from build123d import *

# Parameters (mm, degrees)
PAD009_DEPTH    = 2.8
FILLET004_R     = 0.4
SKETCH025_W     = 12.7
SKETCH025_H     = 1.6
POCKET014_DEPTH = 2.801


with BuildPart() as part:
    # Sketch009 (on Face6 of ShapeBinder008) → Pad009 (new body)
    with BuildSketch(Plane.XZ.offset(60.388718)):
        with BuildLine():
            Line((37.8, 3.127675), (37.8, 0.327675))
            Line((37.8, 0.327675), (23.8, 0.327675))
            ThreePointArc((23.8, 0.327675), (23.4, -0.072325), (23.8, -0.472325))
            Line((23.8, -0.472325), (37.8, -0.472325))
            Line((37.8, -0.472325), (37.8, -33.872325))
            Line((37.8, -33.872325), (23.8, -33.872325))
            ThreePointArc((23.8, -33.872325), (23.4, -34.272325), (23.8, -34.672325))
            Line((23.8, -34.672325), (37.8, -34.672325))
            Line((37.8, -34.672325), (37.8, -37.472325))
            Line((37.8, -37.472325), (35.8, -38.222325))
            Line((35.8, -38.222325), (35.8, -37.472325))
            Line((35.8, -37.472325), (33, -37.472325))
            Line((33, -37.472325), (33, -39.472325))
            Line((33, -39.472325), (25.535898, -37.472325))
            Line((25.535898, -37.472325), (-25.535898, -37.472325))
            Line((-25.535898, -37.472325), (-33, -39.472325))
            Line((-33, -39.472325), (-33, -37.472325))
            Line((-33, -37.472325), (-35.8, -37.472325))
            Line((-35.8, -38.222325), (-35.8, -37.472325))
            Line((-37.8, -37.472325), (-35.8, -38.222325))
            Line((-37.8, -37.472325), (-37.8, -34.672325))
            Line((-37.8, -34.672325), (-23.8, -34.672325))
            ThreePointArc((-23.8, -34.672325), (-23.4, -34.272325), (-23.8, -33.872325))
            Line((-23.8, -33.872325), (-37.8, -33.872325))
            Line((-37.8, -33.872325), (-37.8, -0.472325))
            Line((-37.8, -0.472325), (-23.8, -0.472325))
            ThreePointArc((-23.8, -0.472325), (-23.4, -0.072325), (-23.8, 0.327675))
            Line((-23.8, 0.327675), (-37.8, 0.327675))
            Line((-37.8, 0.327675), (-37.8, 3.127675))
            Line((-37.8, 3.127675), (-35.8, 3.877675))
            Line((-35.8, 3.877675), (-35.8, 3.127675))
            Line((-35.8, 3.127675), (-33, 3.127675))
            Line((-33, 3.127675), (-33, 5.127675))
            Line((-33, 5.127675), (-25.535898, 3.127675))
            Line((-25.535898, 3.127675), (25.535898, 3.127675))
            Line((25.535898, 3.127675), (33, 5.127675))
            Line((33, 5.127675), (33, 3.127675))
            Line((33, 3.127675), (35.8, 3.127675))
            Line((35.8, 3.877675), (35.8, 3.127675))
            Line((37.8, 3.127675), (35.8, 3.877675))
        make_face()
    extrude(amount=-PAD009_DEPTH)

    # Fillet004
    fillet004_edges = [part.edges().sort_by_distance(p)[0] for p in [
        (33, -58.988718, 5.127675),
        (37.8, -58.988718, 3.127675),
        (37.8, -58.988718, 0.327675),
        (37.8, -58.988718, -0.472325),
        (37.8, -58.988718, -33.872325),
        (37.8, -58.988718, -34.672325),
        (37.8, -58.988718, -37.472325),
        (33, -58.988718, -39.472325),
        (-37.8, -58.988718, -33.872325),
        (-37.8, -58.988718, -34.672325),
        (-37.8, -58.988718, -37.472325),
        (-33, -58.988718, -39.472325),
        (-33, -58.988718, 5.127675),
        (-37.8, -58.988718, 3.127675),
        (-37.8, -58.988718, 0.327675),
        (-37.8, -58.988718, -0.472325),
    ]]
    fillet(fillet004_edges, radius=FILLET004_R)

    # Sketch025 (on Face2 of Fillet004) → Pocket014 (cut, through all)
    with BuildSketch(Plane.XZ.offset(60.388718)):
        with Locations((-19.05, -5.472325)):
            Rectangle(SKETCH025_W, SKETCH025_H)
        with Locations((19.05, -5.472325)):
            Rectangle(SKETCH025_W, SKETCH025_H)
    extrude(amount=-POCKET014_DEPTH, mode=Mode.SUBTRACT)


solid = part.part
The listing builds one solid part. Answer for the finished solid, in the listing's coordinates (mm). A direction names the side the tool comes from. Coordinates: 2 decimals unless noted, no trailing zeros. Loops run counter-clockwise (first coordinate to the right, second up) from the corner with the lowest first, then second, coordinate; pieces in that order, holes last. Notation, with made-up numbers: M -31.75,-31.75 L -9.75,-31.75 A19 cw -9.75,-18.75 Z; hole C -7.75,-4 d10. An arc over 180 degrees is marked long. Answer in a Markdown table with one row per item.
1) Given pin 1 (1.5 mm diameter, centred on x = 16.5, y = -60, fed in from +Z); pin 2 (0.8 mm diameter, centred on x = 28.5, y = -58.5, fed in from -Z); pin 3 (1.4 mm diameter, centred on x = -30.5, y = -59, fed in from -Z); pin 4 (0.8 mm diameter, centred on x = -33, y = -59, fed in from +Z), each flat-ended and moving along its own axis, determine where each tip first touches the part or whether it passes through.
Answers below:
| item | result |
|---|---|
| pin 1 | z = 3.13 |
| pin 2 | z = -38.37 |
| pin 3 | z = -38.99 |
| pin 4 | z = 5.01 |
2) Which of the six approach directions +Z, -Z, +X, -X, +Y, -Y give full straight-line access (tool end or side, diameter ignored) to faces 5 (the flat face through (29.065, -59.008, -38.418)), 6 (the flat face through (34, -59, 3.128)), 7 (the flat face through (31, -59, 0.328)), 8 (the flat face through (19, -59, -4.672)), 9 (the flat face through (-36.682, -59.008, -37.891))?
Answers below:
| item | result |
|---|---|
| face 5 | -Z, +Y, -Y |
| face 6 | +Z, +Y, -Y |
| face 7 | +X, +Y, -Y |
| face 8 | +Y, -Y |
| face 9 | -Z, -X, +Y, -Y |
3) Find section B-B (y = -59.55). Count the separate pieces of the cut face and the enclosed holes in it, then the cut area to 3 significant figures.
Answers below:
| item | result |
|---|---|
| separate pieces | 1 |
| enclosed holes | 2 |
| area | 3,020 mm^2 |
4) Find section C-C (x = 3). Determine the outline of the cut face in (y, z).
Answers below:
| item | result |
|---|---|
| outline | M -60.39,-37.47 L -57.59,-37.47 L -57.59,3.13 L -60.39,3.13 Z |
5) Find section A-A (x = 20). Determine the outline of the cut face in (y, z), then the cut area to 3 significant figures.
Answers below:
| item | result |
|---|---|
| outline | M -60.39,-37.47 L -57.59,-37.47 L -57.59,-6.27 L -60.39,-6.27 Z; M -60.39,-4.67 L -57.59,-4.67 L -57.59,3.13 L -60.39,3.13 Z |
| area | 109 mm^2 |
6) Determine the mould class of faces 1 (the flat face through (12.7, -59, -5)), 2 (the flat face through (37.8, -59, -17)), 3 (the flat face through (-31, -59, -34.672)), 4 (the flat face through (-12.7, -59, -5)) for opening direction X: released by +X, released by -X, zero draft, split by the parting line, or undercut.
Answers below:
| item | result |
|---|---|
| face 1 | undercut |
| face 2 | released by +X |
| face 3 | zero draft |
| face 4 | undercut |
7) Find the intervals of material crossed by probe 1 along Z at (x, y) = (-24.5, -59.15); probe 2 along Z at (x, y) = (-31, -58.95); probe 3 along Z at (x, y) = (21.5, -58.3), in increasing order.
Answers below:
| item | result |
|---|---|
| probe 1 | -37.47 to -34.67, -33.87 to -6.27, -4.67 to -0.47, 0.33 to 3.13 |
| probe 2 | -38.94 to -34.67, -33.87 to -0.47, 0.33 to 4.59 |
| probe 3 | -37.47 to -6.27, -4.67 to 3.13 |
